from build123d import *

# Parameters (mm, degrees)
BOSS_EXTRUDE1_DEPTH = 5.35


with BuildPart() as part:
    # Model → Boss-Extrude1 (new body)
    with BuildSketch(Plane.XY):
        with BuildLine():
            Line((23.530324921, 0), (13.730324805, 0))
            Line((13.730324805, 0), (13.730324805, 25.000000373))
            Line((13.730324805, 25.000000373), (8.38032458, 25.000000373))
            Line((8.38032458, 25.000000373), (8.38032458, 1.418154687))
            Line((8.38032458, 1.418154687), (4, 1.418154687))
            ThreePointArc((4, 1.418154687), (1.171572808, 2.589727629), (0, 5.418154877))
            Line((0, 5.418154877), (0, 33.278149277))
            ThreePointArc((0, 33.278149277), (1.171572778, 36.106576304), (3.999999724, 37.278149277))
            Line((3.999999724, 37.278149277), (25.530324042, 37.278149277))
            ThreePointArc((25.530324042, 37.278149277), (28.358750081, 36.106577487), (29.530324042, 33.278152347))
            Line((29.530324042, 33.278152347), (29.530324042, 6))
            ThreePointArc((29.530324042, 6), (27.77296504, 1.757359624), (23.530324921, 0))
        make_face()
    extrude(amount=BOSS_EXTRUDE1_DEPTH)


solid = part.part
Read the model definition and answer for the solid it produces. Units are mm, in the model's axes. A direction names the side the tool comes from. Coordinates: 2 decimals unless noted, no trailing zeros. Loops run counter-clockwise (first coordinate to the right, second up) from the corner with the lowest first, then second, coordinate; pieces in that order, holes last. Notation, with made-up numbers: (20.25, -8) - (28.25, -8) arc R31 cw to (28.25, 26) - close; hole circle Ø5 at (52, -24.75). An arc over 180 degrees is marked (long way). Answer in a Markdown table with one row per item.
Q1. The mould has two halves that part along X. Classify faces 1 (the flat face through (13.73, 12, 3)), 2 (the flat face through (15, 19, 5.35)), 3 (the flat face through (29.53, 20, 3)), 4 (the cylindrical face through (1.141, 36.075, 2.638)): pulls with the +X half, pulls with the -X half, needs draft (parallel to the pull), parting line crosses it, or undercut.
Here are the results:
| item | result |
|---|---|
| face 1 | undercut |
| face 2 | needs draft |
| face 3 | pulls with the +X half |
| face 4 | pulls with the -X half |
Q2. Find section A-A on y = 12.5. Write down the section's boundary in (x, z).
Here are the results:
| item | result |
|---|---|
| outline | (0, 0) - (8.38, 0) - (8.38, 5.35) - (0, 5.35) - close; (13.73, 0) - (29.53, 0) - (29.53, 5.35) - (13.73, 5.35) - close |
Q3. Straight lines are drawn through the part: line 1 along X through (y, z) = (15, 3.05); line 2 along Y through (x, z) = (4.5, 4.25); line 3 along Y through (x, z) = (11, 3.5). For each, find the intervals that lie inside material, in ascending order. Write a range as [from, to].
Here are the results:
| item | result |
|---|---|
| line 1 | x = [0, 8.38], [13.73, 29.53] |
| line 2 | y = [1.42, 37.28] |
| line 3 | y = [25, 37.28] |
Q4. Find section D-D on x = 4.75. Write down the section's boundary in (y, z).
Here are the results:
| item | result |
|---|---|
| outline | (1.42, 0) - (37.28, 0) - (37.28, 5.35) - (1.42, 5.35) - close |
Q5. Find section C-C on x = 12. Write down the section's boundary in (y, z), plus the area to 3 significant figures.
Here are the results:
| item | result |
|---|---|
| outline | (25, 0) - (37.28, 0) - (37.28, 5.35) - (25, 5.35) - close |
| area | 65.7 mm^2 |
Q6. For faces 5 (the flat face through (6, 1.418, 3)), 6 (the flat face through (15, 19, 0)), 7 (the flat face through (11, 25, 3)), determine the directions among +Z, -Z, +X, -X, +Y, -Y from which every point of the face is accessible in a straight line to the end or side of a thin tool.
Here are the results:
| item | result |
|---|---|
| face 5 | +Z, -Z, -X, -Y |
| face 6 | -Z, +X, -X, +Y, -Y |
| face 7 | +Z, -Z, -Y |
Q7. Find section B-B on z = 1.7. Write down the section's boundary in (x, y), plus the area to 3 significant figures.
Here are the results:
| item | result |
|---|---|
| outline | (0, 5.42) arc R4 ccw to (4, 1.42) - (8.38, 1.42) - (8.38, 25) - (13.73, 25) - (13.73, 0) - (23.53, 0) arc R6 ccw to (29.53, 6) - (29.53, 33.28) arc R4 ccw to (25.53, 37.28) - (4, 37.28) arc R4 ccw to (0, 33.28) - close |
| area | 937 mm^2 |
